Design review of the part built by this model. Coordinates are the model's own, in mm. A direction names the side the tool comes from. Coordinates: 2 decimals unless noted, no trailing zeros. Loops run counter-clockwise (first coordinate to the right, second up) from the corner with the lowest first, then second, coordinate; pieces in that order, holes last. Notation, with made-up numbers: (11, -18) - (27, -18) arc R22 ccw to (27, -4) - close; hole circle Ø4 at (63, 76). An arc over 180 degrees is marked (long way). Answer in a Markdown table with one row per item. Add a question column.
(1) For faces 1 (the face through (-12, -28, 20.355)), 2 (the face through (48.827, -50, 0)), 3 (the face through (-48.827, -45, 0)), 4 (the face through (-37.17, -72.72, 0.31)), list the 3-axis set-ups (+Z, -Z, +X, -X, +Y, -Y) from which the entire face can be reached by the end or side of a thin tool; tool diameter is ignored.
(2) We need section C-C, the plane y = -39. Write out the cut boundary in (x, z).
(3) The part is to be moulded in two halves that separate along X. For faces 5 (the face through (101.353, -12.522, -0.621)), 6 (the face through (65.112, -12.878, -16.496)), 7 (the face through (0, -25.4, 23)), say which applies: released by +X, released by -X, zero draft, split by the parting line, or undercut.
(4) We need section A-A, the plane y = -13. Write out the cut boundary in (x, z).
(5) Clearance check with flat-ended pins moving along their axes: pin 1 (19 mm diameter, centred on y = -62.11, z = 0, fed in from +X); pin 2 (1 mm diameter, centred on x = -13, z = -18.5, fed in from -Y); pin 3 (6 mm diameter, centred on y = -14.5, z = 13, fed in from +X); pin 4 (15 mm diameter, centred on x = 16.5, y = -44.5, fed in from +Z). State where each tip first meets the part, or that it passes through.
(6) We need section D-D, the plane x = 0. Write out the cut boundary in (y, z), plus the area to 3 significant figures.
(7) We need section B-B, the plane x = -32.5. Write out the cut boundary in (y, z) (3 decimals), plus the area to 3 significant figures.
(8) To check wall thickness, follow L1, parallel to Y at x = -38.5, z = 0; L2, parallel to X at y = -56, z = 13.5; L3, parallel to X at y = -8.5, z = 12. State the ranges of each line that lie inside material, in increasing order. Write a range as [from, to].
from build123d import *

# Parameters (mm, degrees)
F2_DEPTH  = 25.4
F3_R      = 14.2869829167
F3_R_2    = 15.0362053168
F4_DEPTH  = 25.4
F5_R      = 15.0979548497
F6_DEPTH  = 25.4
F7_R      = 16.8973706764
F8_DEPTH  = 12.7
F9_DEPTH  = 25.4
F10_R     = 15.3471381564
F11_DEPTH = 76.2
F12_DEPTH = 25.4
F13_R     = 16.8651828774
F14_DEPTH = 25.4
F15_W     = 97.6533442736
F15_H     = 40.7104864717
F16_DEPTH = 76.2
F17_R     = 30.5155055684
F18_DEPTH = 25.4
F19_DEPTH = 25.4
F20_R     = 10.6213754379
F21_DEPTH = 50.8
F22_R     = 9.4222372935
F23_DEPTH = 50.8
F24_R     = 9.0371424161
F25_DEPTH = 25.4


with BuildPart() as f2:
    # F1 (on face) → F2 (new body)
    with BuildSketch(Plane.XZ):
        with BuildLine():
            Line((75.9671404958, 32.3720407565), (75.9671404958, 33.3821922541))
            Line((75.9671404958, 33.3821922541), (-75.9671404958, 33.3821922541))
            Line((-75.9671404958, 33.3821922541), (-75.9671404958, 31.6472478295))
            ThreePointArc((-75.9671404958, 31.6472478295), (-98.9936606225, 0), (-75.9671404958, -31.6472478295))
            Line((-75.9671404958, -31.6472478295), (-75.9671404958, -33.3821922541))
            Line((-75.9671404958, -33.3821922541), (75.9671404958, -33.3821922541))
            Line((75.9671404958, -33.3821922541), (75.9671404958, -32.3720407565))
            ThreePointArc((75.9671404958, -32.3720407565), (101.3590356441, 0), (75.9671404958, 32.3720407565))
        make_face()
    extrude(amount=F2_DEPTH)

    # F3 (on Front) → F4 (cut)
    with BuildSketch(Plane.XZ):
        with Locations((-75.3733813763, 0)):
            Circle(F3_R)
        with Locations((76.2721076608, 0)):
            Circle(F3_R_2)
    extrude(amount=-F4_DEPTH, mode=Mode.SUBTRACT)

    # F5 (on Front) → F6 (cut)
    with BuildSketch(Plane.XZ):
        with Locations((74.6077895164, 0)):
            Circle(F5_R)
    extrude(amount=-F6_DEPTH, mode=Mode.SUBTRACT)

    # F7 (on Front) → F8 (cut, symmetric)
    with BuildSketch(Plane.XZ):
        with Locations((68.7745809555, 0)):
            Circle(F7_R)
    extrude(amount=F8_DEPTH, both=True, mode=Mode.SUBTRACT)

    # F0 (on Front) → F9 (cut)
    with BuildSketch(Plane.XZ):
        with BuildLine():
            Line((75.9671404958, 33.3821922541), (-75.9671404958, 33.3821922541))
            Line((-75.9671404958, 33.3821922541), (-75.9671404958, 31.6472478295))
            ThreePointArc((-75.9671404958, 31.6472478295), (-98.9936606225, 0), (-75.9671404958, -31.6472478295))
            Line((-75.9671404958, -31.6472478295), (-75.9671404958, -33.3821922541))
            Line((-75.9671404958, -33.3821922541), (75.9671404958, -33.3821922541))
            Line((75.9671404958, -33.3821922541), (75.9671404958, -32.3720407565))
            ThreePointArc((75.9671404958, -32.3720407565), (101.3590356441, 0), (75.9671404958, 32.3720407565))
            Line((75.9671404958, 32.3720407565), (75.9671404958, 33.3821922541))
        make_face()
    extrude(amount=-F9_DEPTH, mode=Mode.SUBTRACT)

    # F10 (on Front) → F11 (cut)
    with BuildSketch(Plane.XZ):
        with Locations((-71.0009858012, 0)):
            Circle(F10_R)
    extrude(amount=-F11_DEPTH, mode=Mode.SUBTRACT)

    # F12 (cut): a face of the model
    f12_faces = [f2.faces().sort_by_distance(p)[0] for p in [
        (68.7745809555, -12.7, 0),
    ]]
    extrude(f12_faces, amount=-F12_DEPTH, mode=Mode.SUBTRACT)

    # F13 (on face) → F14 (cut)
    with BuildSketch(Plane.XZ.offset(25.4)):
        with Locations((-74.4160786271, 0)):
            Circle(F13_R)
    extrude(amount=-F14_DEPTH, mode=Mode.SUBTRACT)

    # F15 (on Front) → F16 (join)
    with BuildSketch(Plane.XZ):
        Rectangle(F15_W, F15_H)
    extrude(amount=F16_DEPTH)

    # F17 (on Top) → F18 (cut)
    with BuildSketch(Plane.XY):
        with Locations((0, -56.5003752708)):
            Circle(F17_R)
    extrude(amount=-F18_DEPTH, mode=Mode.SUBTRACT)

    # F19 (cut): a face of the model
    f19_faces = [f2.faces().sort_by_distance(p)[0] for p in [
        (0, -53.2237488091, 0),
    ]]
    extrude(f19_faces, amount=-F19_DEPTH, mode=Mode.SUBTRACT)

    # F20 (on Right) → F21 (cut)
    with BuildSketch(Plane.YZ):
        with Locations((-62.1050074697, 0)):
            Circle(F20_R)
    extrude(amount=-F21_DEPTH, mode=Mode.SUBTRACT)

    # F22 (on Right) → F23 (cut)
    with BuildSketch(Plane.YZ):
        with Locations((-58.5186779499, 0)):
            Circle(F22_R)
    extrude(amount=-F23_DEPTH, mode=Mode.SUBTRACT)

    # F24 (on face) → F25 (cut)
    with BuildSketch(Plane.YZ.offset(48.8266721368)):
        with Locations((-64.5882040262, 0)):
            Circle(F24_R)
    extrude(amount=-F25_DEPTH, mode=Mode.SUBTRACT)


solid = f2.part
Responses:
| question | item | result |
|---|---|---|
| 1 | face 1 | +Z, +X, -X, -Y |
| 1 | face 2 | +Z, -Z, +X, -Y |
| 1 | face 3 | +Z, -Z, -X, -Y |
| 1 | face 4 | -X |
| 2 | outline | (-48.83, -20.36) - (-25, -20.36) - (-25, 20.36) - (-48.83, 20.36) - close; (25, -20.36) - (48.83, -20.36) - (48.83, 20.36) - (25, 20.36) - close |
| 3 | face 5 | released by +X |
| 3 | face 6 | undercut |
| 3 | face 7 | zero draft |
| 4 | outline | (-75.97, -33.38) - (75.97, -33.38) - (75.97, -32.37) arc R33.33 ccw to (75.97, 32.37) - (75.97, 33.38) - (-75.97, 33.38) - (-75.97, 31.65) arc R33.26 ccw to (-75.97, -31.65) - close; hole circle Ø33.73 at (-74.42, 0); hole circle Ø33.79 at (68.77, 0) |
| 5 | pin 1 | stops at x = 48.83 |
| 5 | pin 2 | stops at y = -29.13 |
| 5 | pin 3 | stops at x = 99.82 |
| 5 | pin 4 | passes through |
| 6 | outline | (-25.98, -20.36) - (-25.4, -20.36) - (-25.4, -33.38) - (0, -33.38) - (0, 33.38) - (-25.4, 33.38) - (-25.4, 20.36) - (-25.98, 20.36) - close |
| 6 | area | 1,720 mm2 |
| 7 | outline | (-76.2, -20.355) - (-25.4, -20.355) - (-25.4, -33.382) - (0, -33.382) - (0, 33.382) - (-25.4, 33.382) - (-25.4, 20.355) - (-76.2, 20.355) - close; hole (-56.961, -9.293) arc R9.422 ccw to (-56.961, 9.293) arc R10.621 ccw (long way) to start |
| 7 | area | 3,370 mm2 |
| 8 | L1 | y = [-76.2, -72.73], [-49.1, 0] |
| 8 | L2 | x = [-48.83, -30.51], [30.51, 48.83] |
| 8 | L3 | x = [-96.75, -86.27], [-62.57, 56.88], [80.67, 99.12] |
